The listing builds one solid part. Answer for the finished solid, in the listing's coordinates (mm). A direction names the side the tool comes from. Coordinates: 2 decimals unless noted, no trailing zeros. Order: outer loops, then holes, each group sorted by start corner. A loop starts at its lowest first (then second) coordinate and runs counter-clockwise, first axis right, second up. Notation, with made-up numbers: (-29, 8.5) -> (16, 8.5) arc R16 cw to (16, 30.5) -> close; hole circle Ø6 at (40.5, -33). An arc over 180 degrees is marked (long way). Return JSON: item names as keys, results as strings.
```python
from build123d import *

# Parameters (mm, degrees)
F1_DEPTH     = 19
F2_R         = 11
F3_DEPTH     = 19
F5_DEPTH     = 45
F6_W         = 39.6946725957
F6_H         = 17
F7_DEPTH     = 15
F8_W         = 39.6946725957
F8_H         = 16.2631579523
F9_DEPTH     = 30
F10_T1_DEPTH = 39.6946725957
F10_T6_DEPTH = 39.6946725957
F11_W        = 39.6946725957
F11_H        = 16.2631579523
F12_DEPTH    = 45
F13_T4_DEPTH = 39.6946725957


# Not quite as in the source:
# - a fillet or chamfer that OpenCascade refuses, or shapes differently, is made with other operations: its cross-section is extruded or revolved along the edge and cut away or added


with BuildPart() as f1:
    # F0 (on Top) → F1 (new body)
    with BuildSketch(Plane.XY):
        with BuildLine():
            ThreePointArc((-107.8725005202, 54.8863680974), (-139.1356584725, 23.6232101452), (-107.8725005202, -7.6399478071))
            Line((-107.8725005202, -7.6399478071), (6.1274994798, -7.6399478071))
            ThreePointArc((6.1274994798, -7.6399478071), (37.3906574321, 23.6232101452), (6.1274994798, 54.8863680974))
            Line((6.1274994798, 54.8863680974), (-107.8725005202, 54.8863680974))
        make_face()
    extrude(amount=F1_DEPTH)

    # F2 (on face) → F3 (cut)
    with BuildSketch(Plane.XY.offset(19)):
        with Locations((-107.8725005202, 23.6232101452)):
            Circle(F2_R)
        with Locations((6.1274994798, 23.6232101452)):
            Circle(F2_R)
    extrude(amount=-F3_DEPTH, mode=Mode.SUBTRACT)

    # F4 (on face) → F5 (join)
    with BuildSketch(Plane.XY.offset(19)):
        Polygon((-17.1778279245, 54.8863680974), (-82.8725005202, 54.8863680974), (-82.8725005202, -7.6399478071), (-69.8725005202, -7.6399478071), (-69.8725005202, 41.8863680974), (-30.1778279245, 41.8863680974), (-30.1778279245, -7.6399478071), (-17.1778279245, -7.6399478071), align=None)
    extrude(amount=F5_DEPTH)

    # F6 (on face) → F7 (join)
    with BuildSketch(Plane.XY.offset(19)):
        with Locations((-50.0251642223, 0.8600521929)):
            Rectangle(F6_W, F6_H)
    extrude(amount=F7_DEPTH)

    # F8 (on face) → F9 (join)
    with BuildSketch(Plane.XY.offset(19)):
        with Locations((-50.0251642223, 17.491631169)):
            Rectangle(F8_W, F8_H)
    extrude(amount=F9_DEPTH)

    # F10: chamfer of 16 on 2 edges, made by hand

    # F10_s2 → F10_t1 (cut)
    with BuildSketch(Plane.YZ.offset(-69.8725005202)):
        Polygon((-7.6399478071, 18), (8.3600521929, 34), (-7.6399478071, 34), align=None)
    extrude(amount=F10_T1_DEPTH, mode=Mode.SUBTRACT)


with BuildPart() as f10_tool4:
    # F10_s5 → F10_t6 (new body)
    with BuildSketch(Plane.YZ.offset(-69.8725005202)):
        Polygon((9.3600521929, 33), (25.3600521929, 49), (9.3600521929, 49), align=None)
    extrude(amount=F10_T6_DEPTH)

    split(bisect_by=Plane.XY.offset(34), keep=Keep.TOP)


with BuildPart() as f1_1:
    add(f1.part)

    # F10_t3: cut F10_tool4
    add(f10_tool4.part, mode=Mode.SUBTRACT)

    # F11 (on face) → F12 (join)
    with BuildSketch(Plane.XY.offset(19)):
        with Locations((-50.0251642223, 33.7547891213)):
            Rectangle(F11_W, F11_H)
    extrude(amount=F12_DEPTH)

    # F13: chamfer of 17 on 1 edges, made by hand


with BuildPart() as f13_tool2:
    # F13_s3 → F13_t4 (new body)
    with BuildSketch(Plane.YZ.offset(-69.8725005202)):
        Polygon((42.6232101452, 64), (25.6232101452, 47), (25.6232101452, 64), align=None)
    extrude(amount=F13_T4_DEPTH)

    split(bisect_by=Plane.XY.offset(49), keep=Keep.TOP)


with BuildPart() as f1_2:
    add(f1_1.part)

    # F13_t1: cut F13_tool2
    add(f13_tool2.part, mode=Mode.SUBTRACT)


solid = f1_2.part
```
Item 1: The part is cut by section C-C on y = 46.5. Determine the outline of the cut face in (x, z), plus the area to 3 significant figures.
Answer list:
{"outline": "(-129.18, 0) -> (27.44, 0) -> (27.44, 19) -> (-17.18, 19) -> (-17.18, 64) -> (-82.87, 64) -> (-82.87, 19) -> (-129.18, 19) -> close", "area": "5,930 mm2"}
Item 2: The part is cut by section D-D on x = -112. Determine the outline of the cut face in (y, z), plus the area to 3 significant figures.
Answer list:
{"outline": "(-7.37, 0) -> (13.43, 0) -> (13.43, 19) -> (-7.37, 19) -> close; (33.82, 0) -> (54.61, 0) -> (54.61, 19) -> (33.82, 19) -> close", "area": "790 mm2"}
Item 3: The part is cut by section B-B on y = 14.5. Determine the outline of the cut face in (x, z), plus the area to 4 significant figures.
Answer list:
{"outline": "(-137.77, 0) -> (-114.02, 0) -> (-114.02, 19) -> (-137.77, 19) -> close; (-101.73, 0) -> (-0.02, 0) -> (-0.02, 19) -> (-17.18, 19) -> (-17.18, 64) -> (-30.18, 64) -> (-30.18, 38.14) -> (-69.87, 38.14) -> (-69.87, 64) -> (-82.87, 64) -> (-82.87, 19) -> (-101.73, 19) -> close; (12.27, 0) -> (36.03, 0) -> (36.03, 19) -> (12.27, 19) -> close", "area": "4,765 mm2"}
Item 4: Determine the mould class of faces 5 (the flat face through (-50, 54.886, 24)), 6 (the flat face through (-82.873, 24, 41)), 7 (the flat face through (-69.873, 12, 51)), 8 (the flat face through (-17.178, 23, 41)) for opening direction X: pulls with the +X half, pulls with the -X half, needs draft (parallel to the pull), parting line crosses it, or undercut.
Answer list:
{"face 5": "needs draft", "face 6": "pulls with the -X half", "face 7": "undercut", "face 8": "pulls with the +X half"}
Item 5: Flat-ended cylindrical pins translate along their axes: pin 1 (1 mm diameter, centred on y = 20, z = 23, fed in from -X); pin 2 (4 mm diameter, centred on x = -104, y = 8.5, fed in from +Z); pin 3 (1 mm diameter, centred on x = -52, y = 9, fed in from +Z). Find the tip coordinate at first contact, or state that the pin passes through.
Answer list:
{"pin 1": "x = -82.87", "pin 2": "z = 19", "pin 3": "z = 34"}
Item 6: Find the intervals of material crossed by probe 1 along X at (y, z) = (19.5, 49); probe 2 along X at (y, z) = (48, 33.5); probe 3 along X at (y, z) = (18.5, 4.5), in increasing order.
Answer list:
{"probe 1": "-82.87 to -69.87, -30.18 to -17.18", "probe 2": "-82.87 to -17.18", "probe 3": "-138.71 to -117.61, -98.14 to -3.61, 15.86 to 36.97"}
Item 7: Which of the six approach directions +Z, -Z, +X, -X, +Y, -Y give full straight-line access (tool end or side, diameter ignored) to faces 1 (the flat face through (-30.178, 12, 51)), 2 (the cylindrical face through (-139.13, 24.31, 9.37)), 3 (the flat face through (16, 17, 19)), 4 (the flat face through (-118, 17, 19))?
Answer list:
{"face 1": "+Z, -Y", "face 2": "+Z, -Z, -X", "face 3": "+Z, +X, +Y, -Y", "face 4": "+Z, -X, +Y, -Y"}
Item 8: The part is cut by section A-A on x = -42.5. Determine the outline of the cut face in (y, z).
Answer list:
{"outline": "(-7.64, 0) -> (54.89, 0) -> (54.89, 64) -> (42.62, 64) -> (27.62, 49) -> (25.36, 49) -> (10.36, 34) -> (8.36, 34) -> (-7.64, 18) -> close"}
